from build123d import *

# Parameters (mm, degrees)
SKETCH1_W           = 11
SKETCH1_H           = 6.75
SKETCH3_R           = 6.075
BOSS_EXTRUDE1_DEPTH = 7
SKETCH6_W           = 38
SKETCH6_H           = 38
CUT_EXTRUDE1_DEPTH  = 4.6


with BuildPart() as part:
    # Sketch1 → Revolve1 (revolve)
    with BuildSketch(Plane(origin=(0, 0, 0), x_dir=(0, 0, -1), z_dir=(1, 0, 0))):
        with Locations((20.8, 3.375)):
            Rectangle(SKETCH1_W, SKETCH1_H)
    revolve(axis=Axis((0, 0, -26.3), (0, 0, 1)))

    # Sketch2 → Cut-Revolve1 (revolve, cut)
    with BuildSketch(Plane(origin=(0, 0, 0), x_dir=(0, 0, -1), z_dir=(1, 0, 0))):
        Polygon((15.3, 0), (15.3, 6), (15.8415, 5.4585), (24.3, 5.4585), (25.6085, 4.15), (26.3, 4.15), (26.3, 0), align=None)
    revolve(axis=Axis((0, 0, -26.3), (0, 0, 1)), mode=Mode.SUBTRACT)

    # Sketch3 → Boss-Extrude1 (add)
    with BuildSketch(Plane.XY.offset(-19.3)):
        with BuildLine():
            ThreePointArc((-6.461141261, 2.693260775), (-7, 0), (-6.461141261, -2.693260775))
            ThreePointArc((-6.461141261, -2.693260775), (-6.84160069, -3.95), (-5.563002881, -4.248882082))
            ThreePointArc((-5.563002881, -4.248882082), (-3.5, -6.062177826), (-0.898138381, -6.942142857))
            ThreePointArc((-0.898138381, -6.942142857), (0, -7.9), (0.898138381, -6.942142857))
            ThreePointArc((0.898138381, -6.942142857), (3.5, -6.062177826), (5.563002881, -4.248882082))
            ThreePointArc((5.563002881, -4.248882082), (6.84160069, -3.95), (6.461141261, -2.693260775))
            ThreePointArc((6.461141261, -2.693260775), (7, 0), (6.461141261, 2.693260775))
            ThreePointArc((6.461141261, 2.693260775), (6.84160069, 3.95), (5.563002881, 4.248882082))
            ThreePointArc((5.563002881, 4.248882082), (3.5, 6.062177826), (0.898138381, 6.942142857))
            ThreePointArc((0.898138381, 6.942142857), (0, 7.9), (-0.898138381, 6.942142857))
            ThreePointArc((-0.898138381, 6.942142857), (-3.5, 6.062177826), (-5.563002881, 4.248882082))
            ThreePointArc((-5.563002881, 4.248882082), (-6.84160069, 3.95), (-6.461141261, 2.693260775))
        make_face()
        Circle(SKETCH3_R, mode=Mode.SUBTRACT)
    extrude(amount=-BOSS_EXTRUDE1_DEPTH)

    # Sketch4 → Cut-Revolve2 (revolve, cut)
    with BuildSketch(Plane(origin=(0, 0, 0), x_dir=(0, 0, -1), z_dir=(1, 0, 0))):
        Polygon((18.3, 20.5875), (18.3, 7.0875), (19.3, 7.0875), (22.8, 10.5875), (27.3, 6.0875), (27.3, 20.5875), align=None)
    revolve(axis=Axis((0, 0, -27.3), (0, 0, 1)), mode=Mode.SUBTRACT)

    # Sketch5 → Revolve2 (revolve)
    with BuildSketch(Plane(origin=(0, 0, 0), x_dir=(0, 0, -1), z_dir=(1, 0, 0))):
        with BuildLine():
            Line((0, 0), (0, 7.475))
            Line((0, 7.475), (0.856, 8.331))
            Line((0.856, 8.331), (6.8, 8.331))
            Line((6.8, 8.331), (6.8, 9.1641))
            Line((6.8, 9.1641), (9.5, 9.1641))
            Line((9.5, 9.1641), (9.5, 11.4))
            Line((9.5, 11.4), (13.590896534, 11.4))
            Line((13.590896534, 11.4), (14.1, 9.5))
            Line((14.1, 9.5), (14.1, 6.4))
            ThreePointArc((14.1, 6.4), (14.217157288, 6.117157288), (14.5, 6))
            Line((14.5, 6), (20.1, 6))
            Line((20.1, 6), (21.1, 5))
            Line((21.1, 5), (21.1, 3.6))
            ThreePointArc((21.1, 3.6), (21.158578644, 3.458578644), (21.3, 3.4))
            Line((21.3, 3.4), (25, 3.4))
            ThreePointArc((25, 3.4), (25.085169797, 3.587965433), (25.282648033, 3.647859044))
            Line((25.282648033, 3.647859044), (27.2, 2.95))
            Line((27.2, 2.95), (28, 2.95))
            ThreePointArc((28, 2.95), (28.212132034, 2.862132034), (28.3, 2.65))
            Line((28.3, 2.65), (28.3, 0))
            Line((28.3, 0), (0, 0))
        make_face()
    revolve(axis=Axis((0, 0, -28.3), (0, 0, 1)))

    # Sketch6 → Cut-Extrude1 (cut)
    with BuildSketch(Plane.XY.offset(-14.1)):
        Rectangle(SKETCH6_W, SKETCH6_H)
        Polygon((-9.5, 5.484827557), (-9.5, -5.484827557), (0, -10.969655115), (9.5, -5.484827557), (9.5, 5.484827557), (0, 10.969655115), align=None, mode=Mode.SUBTRACT)
    extrude(amount=CUT_EXTRUDE1_DEPTH, mode=Mode.SUBTRACT)

    # Sketch7 → Cut-Revolve3 (revolve, cut)
    with BuildSketch(Plane(origin=(0, 0, 0), x_dir=(0, 0, -1), z_dir=(1, 0, 0))):
        Polygon((0, 0), (0, 3.489230485), (1.8, 2.45), (28.3, 2.45), (28.3, 0), align=None)
    revolve(axis=Axis((0, 0, -28.3), (0, 0, 1)), mode=Mode.SUBTRACT)


solid = part.part
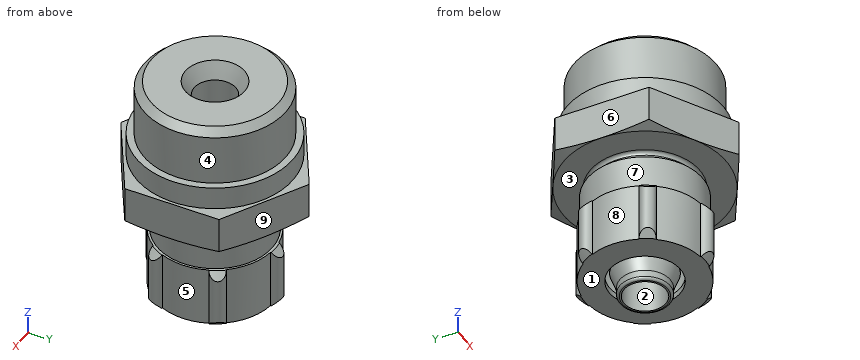
Part model, mm, in its own coordinate system. Face numbers are marked on the shaded views. A direction names the side the tool comes from. Coordinates: 2 decimals unless noted, no trailing zeros. Order: outer loops, then holes, each group sorted by start corner. A loop starts at its lowest first (then second) coordinate and runs counter-clockwise, first axis right, second up.
(1) Probe L1, parallel to X at y = 0, z = -22.9; L2, parallel to Y at x = 0, z = -16.75; L3, parallel to Y at x = 0, z = -25.95. List the from-to ranges inside material, lowest first.
Check sheet entries:
L1: x = -7 to -5.46, -3.4 to -2.45, 2.45 to 3.4, 5.46 to 7
L2: y = -6.75 to -2.45, 2.45 to 6.75
L3: y = -7.44 to -4.15, -3.4 to -2.45, 2.45 to 3.4, 4.15 to 7.44
(2) Pull direction Y, two halves, no side cores. Call the marked faces 6, 7, 8 and 9: pulls with the +Y half, pulls with the -Y half, needs draft (parallel to the pull), parting line crosses it, or undercut.
Check sheet entries:
face 6: needs draft
face 7: parting line crosses it
face 8: undercut
face 9: pulls with the +Y half
(3) Slice it at C-C, the plane z = -8. Write the cut outline in (x, y), and give its area (3 significant figures).
Check sheet entries:
outline: circle Ø18.33 at (0, 0); hole circle Ø4.9 at (0, 0)
area: 245 mm2
(4) Pin check, flat tips, straight feed: pin 1 Ø4 at (x, y) = (7, -0.5) entering from -Z; pin 2 Ø4 at (y, z) = (-3, -3) entering from -X; pin 3 Ø5 at (y, z) = (-8.5, -20.5) entering from -X. Stop position of each tip, or through.
Check sheet entries:
pin 1: stops at z = -26.3
pin 2: stops at x = -8.27
pin 3: stops at x = -3.61
(5) Slice it at B-B, the plane z = -12.25. Write the cut outline in (x, y), and give its area (3 significant figures).
Check sheet entries:
outline: (-9.5, -5.48) - (0, -10.97) - (9.5, -5.48) - (9.5, 5.48) - (0, 10.97) - (-9.5, 5.48) - close; hole circle Ø4.9 at (0, 0)
area: 294 mm2
(6) Slice it at A-A, the plane z = -23. Write the cut outline in (x, y), and give its area (3 significant figures).
Check sheet entries:
outline: (-6.46, -2.69) arc R0.9 ccw (long way) to (-5.56, -4.25) arc R7 ccw to (-0.9, -6.94) arc R0.9 ccw (long way) to (0.9, -6.94) arc R7 ccw to (5.56, -4.25) arc R0.9 ccw (long way) to (6.46, -2.69) arc R7 ccw to (6.46, 2.69) arc R0.9 ccw (long way) to (5.56, 4.25) arc R7 ccw to (0.9, 6.94) arc R0.9 ccw (long way) to (-0.9, 6.94) arc R7 ccw to (-5.56, 4.25) arc R0.9 ccw (long way) to (-6.46, 2.69) arc R7 ccw to start; circle Ø6.8 at (0, 0); hole circle Ø10.92 at (0, 0); hole circle Ø4.9 at (0, 0)
area: 85.6 mm2
(7) Slice it at D-D, the plane z = -5. Write the cut outline in (x, y).
Check sheet entries:
outline: circle Ø16.66 at (0, 0); hole circle Ø4.9 at (0, 0)
(8) Tool access for the marked faces 1, 2, 3, 4 and 5: list every direction of +Z, -Z, +X, -X, +Y, -Y with a clear straight run to the whole face (end or side of a thin tool).
Check sheet entries:
face 1: -Z
face 2: +Z, -Z
face 3: none
face 4: +Z
face 5: -Z, +X
